Autodesk Inventor part; units mm, degrees
ref_plane "YZ Plane" through (0, 0, 0) normal (1, 0, 0) x (0, 1, 0)
ref_plane "XZ Plane" through (0, 0, 0) normal (0, 1, 0) x (-1, 0, 0)
ref_plane "XY Plane" through (0, 0, 0) normal (0, 0, 1) x (1, 0, 0)
sketch "Sketch1" plane through (0, 0, 0) normal (0, 0, 1) x (1, 0, 0)
  line L0 (-136.525, 26.9398) -> (153.9875, -24.2854)
  line L1 (153.9875, -21.0615) -> (153.9875, -24.2854)
  line L2 (153.9875, -21.0615) -> (-136.525, 30.1637)
  line L3 (-136.525, 26.9398) -> (-136.525, 30.1637)
  point P0 (0, 0)
extrude "Extrusion1" add sketch "Sketch1" along normal blind 117.475
hole "Hole1" at (-127.1447, 28.5097, 109.5375) direction (-0.1736, -0.9848, 0) diameter 6.731 depth 25.4 tip angle 118
pattern_linear "Rectangular Pattern1" count 2 spacing 68.2625 along (0, 0, -1) of "Hole1"
pattern_linear "Rectangular Pattern2" count 2 spacing 241.3 along (0.9848, -0.1736, 0) of "Hole1"
properties part number "GE-12086-03"
CAD build for the part. Positions are in the model's coordinates, mm. Round coordinates to 2 decimals unless told otherwise and drop trailing zeros. Write each loop counter-clockwise with the first axis right and the second up, starting at its lowest first coordinate (ties: lowest second). Pieces come first, ordered by that corner, then holes. Notation, with made-up numbers: M 5.5,-14.75 L 37.5,-14.75 A34 cw 37.5,18.25 Z; hole C -22.5,73.5 d5. An arc over 180 degrees is marked long. Put each result on its own line as item: value. Start each with the question number.
1) Pull direction X, two halves, no side cores. Call faces 1 (the cylindrical face through (-128.42, 27.1, 44.485)), 2 (the flat face through (10.765, 4.193, 57.915)), 3 (the flat face through (8, 3, 117.475)): pulls with the +X half, pulls with the -X half, needs draft (parallel to the pull), parting line crosses it, or undercut.
2) Drill centre lines: probe 1 along Y at (x, z) = (62, 23); probe 2 along Y at (x, z) = (117.5, 106). Where is each one in solid material? Low to high. Write a range as [from, to].
3) Saw through at B-B, the plane y = 12.5. Write the cut outline in (x, z) (3 decimals), and give its area (3 significant figures).
4) Saw through at A-A, the plane z = 78. Write the cut outline in (x, y) (1 decimal), and give its area (3 significant figures).
5) Pin check, flat tips, straight feed: pin 1 Ø3 at (x, z) = (97.5, 43.5) entering from -Y; pin 2 Ø8 at (x, z) = (38.5, 27) entering from -Y; pin 3 Ø6 at (x, z) = (-41.5, 50.5) entering from -Y. Stop position of each tip, or through.
Resolved:
1. face 1: undercut
1. face 2: pulls with the +X half
1. face 3: needs draft
2. probe 1: [-8.07, -4.84]
2. probe 2: [-17.85, -14.63]
3. outline: M -54.633,0 L -36.349,0 L -36.349,117.475 L -54.633,117.475 Z
3. area: 2,150 mm²
4. outline: M -136.5,26.9 L 154,-24.3 L 154,-21.1 L -136.5,30.2 Z
4. area: 937 mm²
5. pin 1: y = -14.59
5. pin 2: y = -4.63
5. pin 3: y = 9.66
